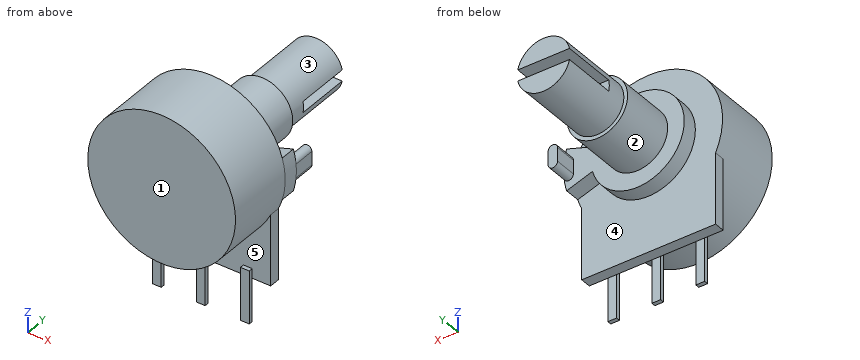
from build123d import *

# Parameters (mm, degrees)
CUT_EXTRUDE1_DEPTH  = 6.2
BOSS_EXTRUDE1_DEPTH = 1.2
SKETCH5_W           = 6
SKETCH5_H           = 0.46
BOSS_EXTRUDE2_DEPTH = 0.5
LPATTERN1_COUNT     = 2
LPATTERN1_PITCH     = 5
LPATTERN1_COL_COUNT = 2
LPATTERN1_COL_PITCH = 5
BOSS_EXTRUDE3_START = 1.76
BOSS_EXTRUDE3_DEPTH = 1.76
BOSS_EXTRUDE4_DEPTH = 2.5


# Read off the part's stored shape, not the designer's step: Boss-Extrude4
with BuildPart() as part:
    # Sketch1 → Revolve1 (revolve)
    with BuildSketch(Plane(origin=(0, 0, 0), x_dir=(0, 0, -1), z_dir=(1, 0, 0))):
        Polygon((0, 0), (-8.39, 0), (-8.39, 7.85), (-5.305, 7.85), (-5.305, 9.61), (-3.425, 9.61), (-3.425, 15.94), (-3, 15.94), (-3, 24.44), (0, 24.44), align=None)
    revolve(axis=Axis((0, 0, 0), (0, -1, 0)))

    # Sketch3 → Cut-Extrude1 (cut)
    with BuildSketch(Plane(origin=(0, 24.44, 0), x_dir=(1, 0, 0), z_dir=(0, 1, 0))):
        with BuildLine():
            Line((-2.933104158, -0.63), (2.933104158, -0.63))
            ThreePointArc((2.933104158, -0.63), (3, 0), (2.933104158, 0.63))
            Line((2.933104158, 0.63), (-2.933104158, 0.63))
            ThreePointArc((-2.933104158, 0.63), (-3, 0), (-2.933104158, -0.63))
        make_face()
    extrude(amount=-CUT_EXTRUDE1_DEPTH, mode=Mode.SUBTRACT)

    # Sketch4 → Boss-Extrude1 (add)
    with BuildSketch(Plane(origin=(0, 7.85, 0), x_dir=(1, 0, 0), z_dir=(0, 1, 0))):
        with BuildLine():
            Line((-7.6, 3.554166569), (-7.6, 11.61))
            Line((-7.6, 11.61), (7.6, 11.61))
            Line((7.6, 11.61), (7.6, 3.554166569))
            ThreePointArc((7.6, 3.554166569), (0, 8.39), (-7.6, 3.554166569))
        make_face()
    extrude(amount=-BOSS_EXTRUDE1_DEPTH)

    # Sketch5 → Boss-Extrude2 (add, symmetric)
    with BuildSketch(Plane(origin=(0, 0, 0), x_dir=(0, 0, -1), z_dir=(1, 0, 0))):
        with Locations((13.52, 6.42)):
            Rectangle(SKETCH5_W, SKETCH5_H)
    boss_extrude2 = extrude(amount=BOSS_EXTRUDE2_DEPTH, both=True)

    # LPattern1: Boss-Extrude2 ×2
    with Locations(*[(i * LPATTERN1_PITCH, 0, 0) for i in range(1, LPATTERN1_COUNT)]):
        add(boss_extrude2)

    # LPattern1 col: Boss-Extrude2 ×2
    with Locations(*[(-i * LPATTERN1_COL_PITCH, 0, 0) for i in range(1, LPATTERN1_COL_COUNT)]):
        add(boss_extrude2)

    # Sketch6 → Boss-Extrude3 (add)
    with BuildSketch(Plane(origin=(0, 7.85, 0), x_dir=(1, 0, 0), z_dir=(0, 1, 0)).offset(BOSS_EXTRUDE3_START)):
        with BuildLine():
            Line((5.119660633, 1.39), (8.05124214, 2.36))
            ThreePointArc((8.05124214, 2.36), (8.39, 0), (8.05124214, -2.36))
            Line((8.05124214, -2.36), (5.119660633, -1.39))
            ThreePointArc((5.119660633, -1.39), (5.305, 0), (5.119660633, 1.39))
        make_face()
    extrude(amount=-BOSS_EXTRUDE3_DEPTH)

    # Boss-Extrude4 outline → Boss-Extrude4 (add)
    with BuildSketch(Plane(origin=(0, 9.61, 0), x_dir=(1, 0, 0), z_dir=(0, 1, 0))):
        with BuildLine():
            ThreePointArc((8.354129219, 0.775), (7.819129219, 1.31), (7.284129219, 0.775))
            Line((7.284129219, 0.775), (7.284129219, -0.775))
            ThreePointArc((7.284129219, -0.775), (7.819129219, -1.31), (8.354129219, -0.775))
            Line((8.354129219, -0.775), (8.354129219, 0.775))
        make_face()
    extrude(amount=BOSS_EXTRUDE4_DEPTH)


solid = part.part
Input: part model. Units: mm. Frame: model coordinates. Face numbers are marked on the shaded views. A direction names the side the tool comes from. Give positions to 0.01 mm unless a question says otherwise; leave off trailing zeros. Order: outer loops, then holes, each group sorted by start corner. A loop starts at its lowest first (then second) coordinate and runs counter-clockwise, first axis right, second up. Notation, with made-up numbers: (56, 32.25) - (115, 32.25) arc R18 cw to (115, 60.25) - close; hole circle Ø3 at (-37, 17.5). An arc over 180 degrees is marked (long way). Answer as a JSON object with one key per item and string values. Group by question number.
Q1. Set-up query: the marked faces 1 and 2. Return all of +Z, -Z, +X, -X, +Y, -Y with unobstructed straight access to the full face (end or side cutting, diameter ignored); none if empty.
Q2. Cut plane C-C, the plane x = 0. Output: boundary loops of the cut face in (y, z) (3 decimals), then the cut area to 3 significant figures.
Q3. Cut plane A-A, the plane y = 10.25. Output: boundary loops of the cut face in (x, z) (3 decimals), then the cut area to 3 significant figures.
Q4. Mould query, pull axis Z, two halves, no side actions, for the marked faces 3, 4 and 5. Classes: pulls with the +Z half, pulls with the -Z half, needs draft (parallel to the pull), parting line crosses it, or undercut.
Q5. Cut plane B-B, the plane z = 0. Output: boundary loops of the cut face in (x, y) (3 decimals).
Q6. Cut plane D-D, the plane y = 17.5. Output: boundary loops of the cut face in (x, z), then the cut area to 3 significant figures.
Q7. First-contact query: pin 1 Ø8.5 at (x, z) = (-1.5, -0.5) entering from +Y; pin 2 Ø1.5 at (y, z) = (9, -6.5) entering from -X; pin 3 Ø8 at (x, z) = (3, -6.5) entering from +Y; pin 4 Ø0.5 at (x, z) = (0, -14.5) entering from +Y. Flat tips, straight axial feed; report the tip coordinate or a pass-through.
Q8. Line query: probe 1 along Y at (x, z) = (-1.25, 3.25); probe 2 along Y at (x, z) = (-4, -7.5); probe 3 along Z at (x, y) = (-2.5, 23.75). Output: solid intervals per line, ascending.
Results:
{
 "1": {"face 1": "+Z, -Z, +X, -X, -Y", "face 2": "+Y"},
 "2": {"outline": "(0, -8.39) - (6.65, -8.39) - (6.65, -10.52) - (6.19, -10.52) - (6.19, -16.52) - (6.65, -16.52) - (6.65, -11.61) - (7.85, -11.61) - (7.85, -5.305) - (9.61, -5.305) - (9.61, -3.425) - (15.94, -3.425) - (15.94, -3) - (24.44, -3) - (24.44, -0.63) - (18.24, -0.63) - (18.24, 0.63) - (24.44, 0.63) - (24.44, 3) - (15.94, 3) - (15.94, 3.425) - (9.61, 3.425) - (9.61, 5.305) - (7.85, 5.305) - (7.85, 8.39) - (0, 8.39) - close", "area": "244 mm^2"},
 "3": {"outline": "circle Ø6.85 at (0, 0); (7.284, -0.775) arc R0.535 ccw to (8.354, -0.775) - (8.354, 0.775) arc R0.535 ccw to (7.284, 0.775) - close", "area": "39.4 mm^2"},
 "4": {"face 3": "parting line crosses it", "face 4": "needs draft", "face 5": "undercut"},
 "5": {"outline": "(-8.39, 0) - (8.39, 0) - (8.39, 9.61) - (8.354, 9.61) - (8.354, 12.11) - (7.284, 12.11) - (7.284, 9.61) - (3.425, 9.61) - (3.425, 15.94) - (3, 15.94) - (3, 18.24) - (-3, 18.24) - (-3, 15.94) - (-3.425, 15.94) - (-3.425, 9.61) - (-5.305, 9.61) - (-5.305, 7.85) - (-8.39, 7.85) - close"},
 "6": {"outline": "circle Ø6 at (0, 0)", "area": "28.3 mm^2"},
 "7": {"pin 1": "y = 24.44", "pin 2": "through", "pin 3": "y = 15.94", "pin 4": "y = 6.65"},
 "8": {"probe 1": "0 to 9.61", "probe 2": "6.65 to 7.85", "probe 3": "-1.66 to -0.63, 0.63 to 1.66"}
}
